```python
from build123d import *

# Parameters (mm, degrees)
F1_DEPTH = 3
F2_R     = 1.5
F3_DEPTH = 10


# Not quite as in the source:
# - a feature names something its author has since deleted; it is built from what else it names


with BuildPart() as f1:
    # F0 (on Top) → F1 (new body)
    with BuildSketch(Plane.XY):
        with BuildLine():
            ThreePointArc((3.25, 74.9241337907), (2.1924432633, 75.1010126169), (1.25, 75.6123960992))
            Line((1.25, 75.6123960992), (1.25, 2.9241337907))
            ThreePointArc((1.25, 2.9241337907), (1.8357864376, 4.338347353), (3.25, 4.9241337907))
            Line((3.25, 4.9241337907), (3.25, 74.9241337907))
        make_face()
        with BuildLine():
            ThreePointArc((3.25, 4.9241337907), (1.8357864376, 4.338347353), (1.25, 2.9241337907))
            ThreePointArc((1.25, 2.9241337907), (1.8357864376, 1.5099202283), (3.25, 0.9241337907))
            Line((3.25, 0.9241337907), (3.25, 4.9241337907))
        make_face()
        with BuildLine():
            ThreePointArc((5.25, 75.6123960992), (4.3075567367, 75.1010126169), (3.25, 74.9241337907))
            Line((3.25, 74.9241337907), (3.25, 4.9241337907))
            ThreePointArc((3.25, 4.9241337907), (4.6642135624, 4.338347353), (5.25, 2.9241337907))
            Line((5.25, 2.9241337907), (5.25, 75.6123960992))
        make_face()
        with BuildLine():
            ThreePointArc((5.25, 2.9241337907), (4.6642135624, 4.338347353), (3.25, 4.9241337907))
            Line((3.25, 4.9241337907), (3.25, 0.9241337907))
            ThreePointArc((3.25, 0.9241337907), (4.6642135624, 1.5099202283), (5.25, 2.9241337907))
        make_face()
        with BuildLine():
            Line((2.25, 79.6102744523), (1.3928571429, 80.8412521623))
            ThreePointArc((1.3928571429, 80.8412521623), (0.0012122742, 78.2628936507), (1.25, 75.6123960992))
            ThreePointArc((1.25, 75.6123960992), (2.1924432633, 75.1010126169), (3.25, 74.9241337907))
            ThreePointArc((3.25, 74.9241337907), (4.3075567367, 75.1010126169), (5.25, 75.6123960992))
            ThreePointArc((5.25, 75.6123960992), (6.4987877258, 78.2628936507), (5.1071428571, 80.8412521623))
            Line((5.1071428571, 80.8412521623), (4.25, 79.6102744523))
            ThreePointArc((4.25, 79.6102744523), (3.25, 76.4241337907), (2.25, 79.6102744523))
        make_face()
    extrude(amount=F1_DEPTH)

    # F2 (on face) → F3 (join)
    with BuildSketch(Plane.XY.offset(3)):
        with Locations((3.25, 2.9241337907)):
            Circle(F2_R)
    extrude(amount=F3_DEPTH)


solid = f1.part
```
Verification items for the finished model (mm, model axes). A direction names the side the tool comes from. Give positions to 0.01 mm unless a question says otherwise; leave off trailing zeros. Order: outer loops, then holes, each group sorted by start corner. A loop starts at its lowest first (then second) coordinate and runs counter-clockwise, first axis right, second up. Notation, with made-up numbers: (61, 3) - (103, 3) arc R17 cw to (103, 9) - close; hole circle Ø2 at (22, 33.5). An arc over 180 degrees is marked (long way). Answer as CSV lines item,"result". Start each with the question number.
Item 1: Section check A-A, the plane z = 5. Record the boundary of the cut face in (x, y).
Item 2: Access from +Z, -Z, +X, -X, +Y, -Y to the whole of each face (thin tool, end or side, straight path). Record for faces 4 (the face through (5.25, 39, 1)), 5 (the face through (4.636, 2.35, 7.93)), 6 (the face through (1.25, 40, 1)).
Item 3: Gauge pin test, flat ends, axial feed: pin 1 (1 mm diameter, centred on x = 2, y = 67.5, fed in from -Z); pin 2 (1.5 mm diameter, centred on x = 3.5, z = 9, fed in from -Y); pin 3 (0.9 mm diameter, centred on y = 48.5, z = 2, fed in from -X); pin 4 (3 mm diameter, centred on y = 24, z = 2, fed in from +X). Record the tip position at first contact, or that the pin passes through.
Item 4: Section check B-B, the plane y = 37. Record the boundary of the cut face in (x, z).
Item 5: Mould release check, pull along X, two halves, no side actions. Record for faces 1 (the face through (1.827, 80.217, 1.479)), 2 (the face through (6.5, 78.2, 1.5)), 3 (the face through (3, 41, 0)): released by +X, released by -X, zero draft, split by the parting line, or undercut.
Item 6: Material ranges on L1, parallel to Y at x = 3.25, z = 2.45; L2, parallel to X at y = 50.5, z = 1.75; L3, parallel to Z at x = 3, y = 51.5, recorded low to high.
Filled in:
1,outline,"circle Ø3 at (3.25, 2.92)"
2,face 4,"+Z, -Z, +X, -Y"
2,face 5,"+Z"
2,face 6,"+Z, -Z, -X, -Y"
3,pin 1,"z = 0"
3,pin 2,"y = 1.42"
3,pin 3,"x = 1.25"
3,pin 4,"x = 5.25"
4,outline,"(1.25, 0) - (5.25, 0) - (5.25, 3) - (1.25, 3) - close"
5,face 1,"undercut"
5,face 2,"released by +X"
5,face 3,"zero draft"
6,L1,"0.92 to 76.42"
6,L2,"1.25 to 5.25"
6,L3,"0 to 3"
